from build123d import *

# Parameters (mm, degrees)
SKETCH_1_R          = 6
EXTRUDE_1_DEPTH     = 155
SKETCH_2_R          = 3
EXTRUDE_2_DEPTH     = 7
CUT_EXTRUDE_START   = 5
SKETCH_3_R          = 3
SKETCH_3_R_2        = 2.85
CUT_EXTRUDE_1_DEPTH = 0.7
SKETCH_4_R          = 4
EXTRUDE_3_DEPTH     = 23
EXTRUDE_START       = 9
SKETCH_5_R          = 3
EXTRUDE_4_DEPTH     = 9
CHAMFER_1_SIZE      = 0.5
SKETCH_6_W          = 9.301869948
SKETCH_6_H          = 8
CUT_EXTRUDE_2_DEPTH = 1


with BuildPart() as part:
    # 草图1 → 凸台-拉伸1 (new, symmetric)
    with BuildSketch(Plane.XY):
        Circle(SKETCH_1_R)
    extrude(amount=EXTRUDE_1_DEPTH, both=True)

    # 草图2 → 凸台-拉伸2 (add)
    with BuildSketch(Plane(origin=(0, 0, -155), x_dir=(-1, 0, 0), z_dir=(0, 0, -1))):
        with Locations(Location((0, 0, 0), (0, 0, 180))):
            Circle(SKETCH_2_R)
    extrude(amount=EXTRUDE_2_DEPTH)

    # 草图3 → 切除-拉伸1 (cut)
    with BuildSketch(Plane(origin=(0, 0, -155), x_dir=(-1, 0, 0), z_dir=(0, 0, -1)).offset(CUT_EXTRUDE_START)):
        with Locations(Location((0, 0, 0), (0, 0, 180))):
            Circle(SKETCH_3_R)
        Circle(SKETCH_3_R_2, mode=Mode.SUBTRACT)
    extrude(amount=CUT_EXTRUDE_1_DEPTH, mode=Mode.SUBTRACT)

    # 草图4 → 凸台-拉伸3 (add)
    with BuildSketch(Plane.XY.offset(155)):
        Circle(SKETCH_4_R)
    extrude(amount=EXTRUDE_3_DEPTH)

    # 草图5 → 凸台-拉伸4 (add)
    with BuildSketch(Plane.XY.offset(178).offset(EXTRUDE_START)):
        Circle(SKETCH_5_R)
    extrude(amount=-EXTRUDE_4_DEPTH)

    # 倒角1
    chamfer_1_edges = [part.edges().sort_by_distance(p)[0] for p in [
        (-6, 0, -155),
        (-3, 0, 187),
        (-6, 0, 155),
        (-3, 0, -162),
    ]]
    chamfer(chamfer_1_edges, length=CHAMFER_1_SIZE)

    # 草图6 → 切除-拉伸2 (cut)
    with BuildSketch(Plane(origin=(0, 6, 0), x_dir=(1, 0, 0), z_dir=(0, 1, 0))):
        with Locations((0, -146)):
            Rectangle(SKETCH_6_W, SKETCH_6_H)
    cut_extrude_2 = extrude(amount=-CUT_EXTRUDE_2_DEPTH, mode=Mode.SUBTRACT)

    # 镜向1: 切除-拉伸2 across plane
    add(cut_extrude_2.mirror(Plane.ZX), mode=Mode.SUBTRACT)


solid = part.part
Can you work these out from the model? Positions are in its coordinate system, mm. A direction names the side the tool comes from. Give positions to 0.01 mm unless a question says otherwise; leave off trailing zeros. Write each loop counter-clockwise with the first axis right and the second up, starting at its lowest first coordinate (ties: lowest second). Pieces come first, ordered by that corner, then holes. Notation, with made-up numbers: (-0.5, 82.25) -> (12.5, 82.25) arc R25 ccw to (12.5, 119.25) -> close; hole circle Ø4 at (19, -8). An arc over 180 degrees is marked (long way). Answer as a JSON object with one key per item and string values. Group by question number.
Item 1: I'm going to push flat-ended pins straight in: P1, Ø5, axis at y = -3.5, z = -72.5, coming from the +X side; P2, Ø4, axis at x = -4.5, y = -1.5, coming from the +Z side; P3, Ø4, axis at y = -2.5, z = -77.5, coming from the +X side. Where does each tip first touch, or does it pass through?
Item 2: Please list where these lines run through material, in increasing order: line 1 (X direction, y = -3.25, z = 53); line 2 (Y direction, x = -0.5, z = -126); line 3 (X direction, y = 2.25, z = -114). Write a range as [from, to].
Item 3: For faces 1 (the face through (-0.867, -3.905, 166.339)), 2 (the face through (0, -5, 146)), 3 (the face through (-6, 0, 2)), which set-ups out of +Z, -Z, +X, -X, +Y, -Y let a thin tool reach every point of the face, with its end or its side?
Item 4: Suppose I cut it at B-B (z = -16). Please give me the cut outline in (x, y), plus the area to 3 significant figures.
Item 5: We'd pull the mould along Z, two halves only. Please class faces 4 (the face through (0, 5, 146)), 5 (the face through (1, 3, 178)), 6 (the face through (2.4, -2.4, -155)): +Z half, -Z half, draft (parallel to the pull), parting line (faces both ways), or undercut.
Findings:
{
 "1": {"P1": "stops at x = 5.92", "P2": "stops at z = 186.76", "P3": "stops at x = 5.98"},
 "2": {"line 1": "x = [-5.04, 5.04]", "line 2": "y = [-5.98, 5.98]", "line 3": "x = [-5.56, 5.56]"},
 "3": {"face 1": "+Z", "face 2": "+X, -X, -Y", "face 3": "+Z, -Z"},
 "4": {"outline": "circle Ø12 at (0, 0)", "area": "113 mm²"},
 "5": {"face 4": "undercut", "face 5": "+Z half", "face 6": "-Z half"}
}
